Source: CAD feature listing. Evaluate the final solid. Frame: model axes, mm. Coordinates: 2 decimals unless noted, no trailing zeros. Write each loop counter-clockwise with the first axis right and the second up, starting at its lowest first coordinate (ties: lowest second). Pieces come first, ordered by that corner, then holes. Notation, with made-up numbers: M 29.5,-15.75 L 79.5,-15.75 A20 cw 79.5,14.25 Z; hole C 39.25,40 d3. An arc over 180 degrees is marked long. Write item = value, one per line. Start each with the question number.
1. Line query: line 1 along Z through (x, y) = (2.4, 24); line 2 along Z through (x, y) = (2.2, 5.75); line 3 along Y through (x, z) = (0.2, 37). Output: solid intervals per line, ascending.
2. Section query B-B (z = -160). Output: boundary loops of the cut face in (x, y).
3. Pin query (flat end, axial travel): pin 1 Ø1.5 at (x, z) = (2, -13.5) entering from -Y; pin 2 Ø1.5 at (x, z) = (2, 0) entering from -Y; pin 3 Ø1.5 at (x, z) = (2, -11) entering from +Y. Return the tip coordinate at first contact, or that it passes through.
4. Section query A-A (z = 43.5). Output: boundary loops of the cut face in (x, y).
Autodesk Inventor part; units mm, degrees
ref_plane "YZ Plane" through (0, 0, 0) normal (1, 0, 0) x (0, 1, 0)
ref_plane "XZ Plane" through (0, 0, 0) normal (0, 1, 0) x (-1, 0, 0)
ref_plane "XY Plane" through (0, 0, 0) normal (0, 0, 1) x (1, 0, 0)
sketch "Sketch1" plane through (0, 0, 0) normal (1, 0, 0) x (0, 1, 0)
  line L0 (0, 175) -> (30, 175)
  line L1 (30, 175) -> (30, -175)
  line L2 (30, -175) -> (0, -175)
  line L3 (0, -175) -> (0, 175)
  line L4 (30, 50) -> (20, 50)
  line L5 (20, 50) -> (20, -50)
  line L6 (20, -50) -> (30, -50)
  line L7 (30, -50) -> (30, 50)
  point P0 (0, 0)
  point P1 (0, 0)
  point P2 (20, 0)
  dimension "d0" = 30
  dimension "d1" = 350
  dimension "d2" = 0
  dimension "d3" = 100
  dimension "d4" = 0
  dimension "d5" = 10
extrude "Extrusion1" add sketch "Sketch1" along normal blind 3 contours L0 L1 L4 L5 L6 L2 L3
sketch "Sketch2" plane through (3, 0, 0) normal (1, 0, 0) x (0, 0, -1)
  line L0 (-1.55, -10) -> (1.55, -10)
  line L1 (1.55, 0) -> (1.55, 10)
  line L2 (1.55, 10) -> (-1.55, 10)
  line L3 (-1.55, 10) -> (-1.55, 0)
  line L4 (-1.55, -10) -> (1.55, 10) construction
  line L5 (1.55, -10) -> (-1.55, 10) construction
  line L6 (-175, 0) -> (175, 0)
  line L7 (175, 0) -> (175, 30)
  line L8 (175, 30) -> (50, 30)
  line L9 (50, 30) -> (50, 20)
  line L10 (50, 20) -> (-50, 20)
  line L11 (-50, 20) -> (-50, 30)
  line L12 (-50, 30) -> (-175, 30)
  line L13 (-175, 30) -> (-175, 0)
  point P0 (0, 0)
  dimension "d8" = 3.1
  dimension "d9" = 20
extrude "Extrusion2" cut sketch "Sketch2" against normal blind 3 contours L6 L3 L2 L1
sketch "Sketch3" plane through (3, 0, 0) normal (1, 0, 0) x (0, 0, -1)
  line L0 (-50, 30) -> (-175, 30)
  circle A0 centre (-160, 30) radius 5
  circle A1 centre (-145, 30) radius 5
  circle A2 centre (-130, 30) radius 5
  circle A3 centre (-115, 30) radius 5
  circle A4 centre (-85, 30) radius 5
  circle A5 centre (-100, 30) radius 5
  line L1 (-175, 30) -> (-175, 0)
  circle A6 centre (-70, 30) radius 5
  point P0 (0, 0)
  point P1 (-75, 30)
  point P2 (-65, 30)
  point P3 (-90, 30)
  point P4 (-80, 30)
  point P5 (-105, 30)
  point P6 (-95, 30)
  point P7 (-120, 30)
  point P8 (-110, 30)
  point P9 (-135, 30)
  point P10 (-125, 30)
  point P11 (-150, 30)
  point P12 (-140, 30)
  point P13 (-165, 30)
  point P14 (-155, 30)
  dimension "d12" = 10
  dimension "d13" = 10
  dimension "d14" = 10
  dimension "d16" = 10
  dimension "d17" = 10
  dimension "d18" = 10
  dimension "d19" = 15
  dimension "d20" = 15
  dimension "d21" = 15
  dimension "d22" = 15
  dimension "d23" = 15
  dimension "d24" = 15
  dimension "d25" = 10
  dimension "d26" = 15
extrude "Extrusion3" cut sketch "Sketch3" against normal blind 3 contours A6 L0 | A0 L0 | A1 L0 | A2 L0 | A3 L0 | A5 L0 | A4 L0 picked at (-68.8623, 27.8538) picked at (-161.4384, 28.1203) picked at (-146.4384, 28.1203) picked at (-131.2475, 28.8948) picked at (-113.8623, 27.8538) picked at (-98.8623, 27.8538) picked at (-83.8623, 27.8538)
fillet "Fillet1" radius 5 1 edges at (1.5, 30, 175)
fillet "Fillet2" radius 5 1 edges at (1.5, 30, 50)
mirror "Mirror1" about plane through (0, 0, 0) normal (0, 0, 1) of "Extrusion3", "Fillet1", "Fillet2"
sketch "Sketch6" plane through (0, 0, 1.55) normal (0, -1, 0) x (1, 0, 0)
  line L0 (0, 0) -> (3, 0)
  line L1 (3, 173.45) -> (3, 0)
  line L2 (0, 173.45) -> (3, 173.45)
  line L3 (0, 173.45) -> (0, 0)
  line L4 (3, -3.1) -> (0, -3.1)
  line L5 (0, -3.1) -> (0, -176.55)
  line L6 (0, -176.55) -> (3, -176.55)
  line L7 (3, -3.1) -> (3, -176.55)
  line L8 (0, 142.0785) -> (3, 139.0785)
  line L9 (0, 137.8358) -> (3, 134.8358)
  line L10 (0, -137.9358) -> (3, -140.9358)
  line L11 (0, -142.1785) -> (3, -145.1785)
  line L12 (3, 0) -> (3, -3.1)
  line L13 (0, -1.55) -> (3, -1.55)
  point P0 (1.5, -1.55)
  dimension "d42" = 45
  dimension "d43" = 3
  dimension "d44" = 3
  dimension "d45" = 195
  dimension "d50" = 97.5
extrude "Extrusion5" cut sketch "Sketch6" against normal blind 2 contours L3 L8 L1 L9 | L7 L11 L5 L10
equation "\"d13\" = d12"
equation "\"d14\" = d12"
equation "\"d16\" = d12"
equation "\"d17\" = d12"
equation "\"d18\" = d12"
equation "\"d21\" = d20"
equation "\"d22\" = d21"
equation "\"d23\" = d22"
equation "\"d24\" = d23"
equation "\"d25\" = d12"
equation "\"d26\" = d24"
properties part number "StoveTop1" material "Steel"
Results are:
q1.line_1 = -175 to -50, 50 to 175
q1.line_2 = -175 to -1.55, 1.55 to 175
q1.line_3 = 0 to 20
q2.outline = M 0,0 L 3,0 L 3,25 L 0,25 Z
q3.pin_1 = 0
q3.pin_2 = 10
q3.pin_3 = 20
q4.outline = M 0,0 L 3,0 L 3,20 L 0,20 Z
